Geometry: final body of the model. Coordinates: model frame, mm. A direction names the side the tool comes from. Give positions to 0.01 mm unless a question says otherwise; leave off trailing zeros. Write each loop counter-clockwise with the first axis right and the second up, starting at its lowest first coordinate (ties: lowest second). Pieces come first, ordered by that corner, then holes.
Q1. Reachability of faces 1 (the face through (28, 15, 17)), 2 (the face through (28.795, 23.124, 5.479)), 3 (the face through (12, -12, 17)), 4 (the face through (-31, -12, 12)) from +Z, -Z, +X, -X, +Y, -Y: full face, straight path, thin tool, end or side. Return the list, or none.
Q2. Pin query (flat end, axial travel): pin 1 (1.8 mm diameter, centred on y = -6.5, z = 14.5, fed in from -X); pin 2 (0.7 mm diameter, centred on x = -30.5, y = -13, fed in from +Z); pin 3 (0.9 mm diameter, centred on x = -25.5, z = 5.5, fed in from -Y). Return the tip coordinate at first contact, or that it passes through.
Q3. Cut plane A-A on x = 35.4. Return the cut outline in (y, z).
Q4. Cut plane B-B on y = 18.85. Return the cut outline in (x, z).
Q5. Cut plane C-C on z = 5.5. Count the separate pieces of the cut face and the enclosed holes in it, plus the area to 3 significant figures.
Q6. Draft query along Z for faces 5 (the face through (10, -14, 6)), 6 (the face through (-31, 25, 12)), 7 (the face through (22.705, 26.576, 5.479)), 8 (the face through (26, 25, 10)). Return one class per face: pulls with the +Z half, pulls with the -Z half, needs draft (parallel to the pull), parting line crosses it, or undercut.
Q7. Cut plane D-D on x = 0. Return the cut outline in (y, z).
Q8. Line query: L1, parallel to Y at x = -25, z = 5.75; L2, parallel to Y at x = 25.75, z = 3.05; L3, parallel to Z at x = -21, y = -14. Output: solid intervals per line, ascending.
```python
from build123d import *

# Parameters (mm, degrees)
SKETCH_1_R          = 1.5
EXTRUDE_1_DEPTH     = 18
SKETCH_9_W          = 60
SKETCH_9_H          = 18
EXTRUDE_4_DEPTH     = 6
FILLET_1_R          = 5
EXTRUDE_START       = -4
SKETCH_2_R          = 3
SKETCH_2_R_2        = 1.5
EXTRUDE_2_DEPTH     = 4
SKETCH_3_R          = 1.5
CUT_EXTRUDE_1_DEPTH = 8
EXTRUDE_3_REACH     = 48.414
SKETCH_5_W          = 20
SKETCH_5_H          = 20
SKETCH_6_R          = 1.5
CUT_EXTRUDE_6_DEPTH = 8
CUT_EXTRUDE_7_DEPTH = 6
CUT_EXTRUDE_START   = -4
CUT_EXTRUDE_8_DEPTH = 3
SKETCH_10_R         = 5.65
SKETCH_10_R_2       = 4.041451884
EXTRUDE_5_DEPTH     = 12
SKETCH_11_R         = 2
CUT_EXTRUDE_9_DEPTH = 10


with BuildPart() as part:
    # Эскиз1 → Бобышка-Вытянуть1 (new body)
    with BuildSketch(Plane.XY):
        with BuildLine():
            Line((10, -17.8), (30, -17.8))
            Line((30, -17.8), (30, 24.5))
            Line((30, 24.5), (-30, 24.5))
            Line((-30, 24.5), (-30, -17.8))
            Line((-30, -17.8), (-10, -17.8))
            Line((-10, -17.8), (-10, -9.648461447))
            ThreePointArc((-10, -9.648461447), (0, 19.75), (10, -9.648461447))
            Line((10, -9.648461447), (10, -17.8))
        make_face()
        with Locations((-15.5, -12.15)):
            Circle(SKETCH_1_R, mode=Mode.SUBTRACT)
        with Locations((15.5, -12.15)):
            Circle(SKETCH_1_R, mode=Mode.SUBTRACT)
        with Locations((-15.5, 18.85)):
            Circle(SKETCH_1_R, mode=Mode.SUBTRACT)
        with Locations((15.5, 18.85)):
            Circle(SKETCH_1_R, mode=Mode.SUBTRACT)
    extrude(amount=EXTRUDE_1_DEPTH)

    # Эскиз9 → Бобышка-Вытянуть4 (add)
    with BuildSketch(Plane(origin=(0, 24.5, 0), x_dir=(1, 0, 0), z_dir=(0, 1, 0))):
        with Locations((0, -9)):
            Rectangle(SKETCH_9_W, SKETCH_9_H)
    extrude(amount=EXTRUDE_4_DEPTH)

    # Скругление1
    # the kernel refuses this fillet: 5 mm, written as the material it takes off along each edge
    with BuildSketch(Plane(origin=(10, 2.851538553, 18), x_dir=(1, 0, 0), z_dir=(0, -1, 0)), Plane(origin=(-10, -30.3, 18), x_dir=(-1, 0, 0), z_dir=(0, 1, 0))) as fillet_1_piece_1:
        with BuildLine():
            CenterArc((FILLET_1_R, -FILLET_1_R), FILLET_1_R, 90, 90)
            Line((0, -FILLET_1_R), (0, 0))
            Line((0, 0), (FILLET_1_R, 0))
        make_face()
    extrude(amount=33.151538553, mode=Mode.SUBTRACT)
    with BuildSketch(Plane(origin=(30, -30.3, 18), x_dir=(-1, 0, 0), z_dir=(0, 1, 0)), Plane(origin=(-30, 43, 18), x_dir=(1, 0, 0), z_dir=(0, -1, 0))) as fillet_1_piece_2:
        with BuildLine():
            CenterArc((FILLET_1_R, -FILLET_1_R), FILLET_1_R, 90, 90)
            Line((0, -FILLET_1_R), (0, 0))
            Line((0, 0), (FILLET_1_R, 0))
        make_face()
    extrude(amount=73.3, mode=Mode.SUBTRACT)

    # Эскиз2 → Бобышка-Вытянуть2 (add)
    # profile 1 of 2: a face of its own
    with BuildSketch(Plane.XY.offset(18).offset(EXTRUDE_START)):
        with Locations((-15.5, -12.15)):
            Circle(SKETCH_2_R)
        with Locations((-15.5, -12.15)):
            Circle(SKETCH_2_R_2, mode=Mode.SUBTRACT)
    # profile 2 of 2: a face of its own
    with BuildSketch(Plane.XY.offset(18).offset(EXTRUDE_START)):
        with Locations((15.5, -12.15)):
            Circle(SKETCH_2_R)
        with Locations((15.5, -12.15)):
            Circle(SKETCH_2_R_2, mode=Mode.SUBTRACT)
    extrude(amount=EXTRUDE_2_DEPTH)

    # Эскиз3 → Вырез-Вытянуть1 (cut)
    with BuildSketch(Plane.XZ.offset(17.8)):
        with Locations(Location((-21, 12.5, 0), (0, 0, 270))):
            Circle(SKETCH_3_R)
        with Locations(Location((21, 12.5, 0), (0, 0, 270))):
            Circle(SKETCH_3_R)
    extrude(amount=-CUT_EXTRUDE_1_DEPTH, mode=Mode.SUBTRACT)

    # Бобышка-Вытянуть3: up to this face of the body (flat: up to its plane)
    extrude_3_end = Plane(part.part.faces().sort_by_distance((0, 20.520252556, 0))[0])
    # Эскиз5 → Бобышка-Вытянуть3 (add, up to the picked face)
    with BuildSketch(Plane.XY.offset(18), mode=Mode.PRIVATE) as extrude_3_sk1:
        with Locations((30.5, -9.5)):
            Rectangle(SKETCH_5_W, SKETCH_5_H)
    extrude_3_tool1 = split(extrude(extrude_3_sk1.sketch, amount=-EXTRUDE_3_REACH, mode=Mode.PRIVATE), bisect_by=extrude_3_end, keep=Keep.BOTH, mode=Mode.PRIVATE)
    add(extrude_3_tool1.solids().sort_by(Axis((30.5, -9.5, 18), (0, 0, -1)))[0])

    # Эскиз6 → Вырез-Вытянуть6 (cut)
    with BuildSketch(Plane.XZ.offset(17.8)):
        with Locations(Location((21, 12.5, 0), (0, 0, 270))):
            Circle(SKETCH_6_R)
    extrude(amount=-CUT_EXTRUDE_6_DEPTH, mode=Mode.SUBTRACT)

    # Эскиз7 → Вырез-Вытянуть7 (cut)
    with BuildSketch(Plane.XY.offset(18)):
        with BuildLine():
            Line((24.9, -10.485784196), (24.9, -3.485784196))
            ThreePointArc((24.9, -3.485784196), (25.9, -2.485784196), (26.9, -3.485784196))
            Line((26.9, -3.485784196), (26.9, -10.485784196))
            ThreePointArc((26.9, -10.485784196), (25.9, -11.485784196), (24.9, -10.485784196))
        make_face()
        with BuildLine():
            Line((34.4, -10.485784196), (34.4, -3.485784196))
            ThreePointArc((34.4, -3.485784196), (35.4, -2.485784196), (36.4, -3.485784196))
            Line((36.4, -3.485784196), (36.4, -10.485784196))
            ThreePointArc((36.4, -10.485784196), (35.4, -11.485784196), (34.4, -10.485784196))
        make_face()
    extrude(amount=-CUT_EXTRUDE_7_DEPTH, mode=Mode.SUBTRACT)

    # Эскиз8 → Вырез-Вытянуть8 (cut)
    with BuildSketch(Plane(origin=(0, 0, 0), x_dir=(-1, 0, 0), z_dir=(0, 0, -1)).offset(CUT_EXTRUDE_START)):
        Polygon((29.791451884, -11.8), (27.770725942, -8.3), (23.729274058, -8.3), (21.708548116, -11.8), (23.729274058, -15.3), (27.770725942, -15.3), align=None)
        Polygon((-21.708548116, -11.8), (-23.729274058, -8.3), (-27.770725942, -8.3), (-29.791451884, -11.8), (-27.770725942, -15.3), (-23.729274058, -15.3), align=None)
        Polygon((-21.708548116, 24.85), (-23.729274058, 28.35), (-27.770725942, 28.35), (-29.791451884, 24.85), (-27.770725942, 21.35), (-23.729274058, 21.35), align=None)
        Polygon((29.791451884, 24.85), (27.770725942, 28.35), (23.729274058, 28.35), (21.708548116, 24.85), (23.729274058, 21.35), (27.770725942, 21.35), align=None)
    extrude(amount=-CUT_EXTRUDE_8_DEPTH, mode=Mode.SUBTRACT)

    # Эскиз10 → Бобышка-Вытянуть5 (add)
    # profile 1 of 4: a face of its own
    with BuildSketch(Plane(origin=(0, 0, 0), x_dir=(-1, 0, 0), z_dir=(0, 0, -1))):
        with Locations((25.75, -11.8)):
            Circle(SKETCH_10_R)
        with Locations((25.75, -11.8)):
            Circle(SKETCH_10_R_2, mode=Mode.SUBTRACT)
    # profile 2 of 4: a face of its own
    with BuildSketch(Plane(origin=(0, 0, 0), x_dir=(-1, 0, 0), z_dir=(0, 0, -1))):
        with Locations((25.75, 24.85)):
            Circle(SKETCH_10_R)
        with Locations((25.75, 24.85)):
            Circle(SKETCH_10_R_2, mode=Mode.SUBTRACT)
    # profile 3 of 4: a face of its own
    with BuildSketch(Plane(origin=(0, 0, 0), x_dir=(-1, 0, 0), z_dir=(0, 0, -1))):
        with Locations((-25.75, 24.85)):
            Circle(SKETCH_10_R)
        with Locations((-25.75, 24.85)):
            Circle(SKETCH_10_R_2, mode=Mode.SUBTRACT)
    # profile 4 of 4: a face of its own
    with BuildSketch(Plane(origin=(0, 0, 0), x_dir=(-1, 0, 0), z_dir=(0, 0, -1))):
        with Locations((-25.75, -11.8)):
            Circle(SKETCH_10_R)
        with Locations((-25.75, -11.8)):
            Circle(SKETCH_10_R_2, mode=Mode.SUBTRACT)
    extrude(amount=-EXTRUDE_5_DEPTH)

    # Эскиз11 → Вырез-Вытянуть9 (cut)
    with BuildSketch(Plane(origin=(0, 0, 0), x_dir=(-1, 0, 0), z_dir=(0, 0, -1))):
        with Locations((-25.75, 24.85)):
            Circle(SKETCH_11_R)
        with Locations((25.75, 24.85)):
            Circle(SKETCH_11_R)
        with Locations((25.75, -11.8)):
            Circle(SKETCH_11_R)
        with Locations((-25.75, -11.8)):
            Circle(SKETCH_11_R)
    extrude(amount=-CUT_EXTRUDE_9_DEPTH, mode=Mode.SUBTRACT)


solid = part.part
```
Data:
1. face 1: +Z, +X, +Y
1. face 2: none
1. face 3: +Z
1. face 4: +Z, -X, +Y, -Y
2. pin 1: stops at x = -29.96
2. pin 2: stops at z = 12
2. pin 3: stops at y = -17.8
3. outline: (-19.5, 0) - (0.5, 0) - (0.5, 18) - (-2.49, 18) - (-2.49, 12) - (-11.49, 12) - (-11.49, 18) - (-19.5, 18) - close
4. outline: (-30, 0) - (-17, 0) - (-17, 18) - (-25, 18) arc R5 ccw to (-30, 13) - close; (-14, 0) - (-5.36, 0) - (-5.36, 18) - (-14, 18) - close; (5.36, 0) - (14, 0) - (14, 18) - (5.36, 18) - close; (17, 0) - (30, 0) - (30, 13) arc R5 ccw to (25, 18) - (17, 18) - close
5. separate pieces: 1
5. enclosed holes: 8
5. area: 1,990 mm2
6. face 5: needs draft
6. face 6: pulls with the +Z half
6. face 7: undercut
6. face 8: pulls with the -Z half
7. outline: (19.75, 0) - (30.5, 0) - (30.5, 18) - (19.75, 18) - close
8. L1: y = -17.8 to -15.3, -8.3 to 21.35, 28.35 to 30.5
8. L2: y = -19.5 to -13.8, -9.8 to 22.85, 26.85 to 30.5
8. L3: z = 0 to 12, 14 to 18
